Geometry: final body of the model. Coordinates: model frame, mm. A direction names the side the tool comes from. Give positions to 0.01 mm unless a question says otherwise; leave off trailing zeros. Loops run counter-clockwise (first coordinate to the right, second up) from the corner with the lowest first, then second, coordinate; pieces in that order, holes last. Notation, with made-up numbers: (60.25, 78) - (98.25, 78) arc R21 cw to (98.25, 112) - close; hole circle Ø7 at (18.25, -18). An arc over 180 degrees is marked (long way). Answer in a Markdown table with one row per item.
from build123d import *

# Parameters (mm, degrees)
SKETCH1_R           = 5
BOSS_EXTRUDE1_DEPTH = 6.5


with BuildPart() as part:
    # Sketch1 → Boss-Extrude1 (new body)
    with BuildSketch(Plane.XY):
        Polygon((0, -9.814954576), (8.5, -4.907477288), (8.5, 4.907477288), (0, 9.814954576), (-8.5, 4.907477288), (-8.5, -4.907477288), align=None)
        with Locations(Location((0, 0, 0), (0, 0, 180))):
            Circle(SKETCH1_R, mode=Mode.SUBTRACT)
    extrude(amount=BOSS_EXTRUDE1_DEPTH)

    # Sketch3 → Revolve1 (revolve)
    with BuildSketch(Plane(origin=(0, 0, 0), x_dir=(0, 0, -1), z_dir=(0, 1, 0))):
        with BuildLine():
            Line((-6.5, 8.5), (-8.8, 8.5))
            ThreePointArc((-8.8, 8.5), (-9.648528137, 8.148528137), (-10, 7.3))
            Line((-10, 7.3), (-10, 5))
            Line((-10, 5), (-6.5, 5))
            Line((-6.5, 5), (-6.5, 8.5))
        make_face()
    revolve(axis=Axis((0, 0, 0), (0, 0, 1)))

    # Sketch2 → Cut-Revolve1 (revolve, cut)
    with BuildSketch(Plane(origin=(0, 0, 0), x_dir=(0, 0, -1), z_dir=(1, 0, 0)), mode=Mode.PRIVATE) as cut_revolve1_sk:
        Polygon((-6.5, 9.814954576), (-6.5, 8.5), (-5.958333333, 9.814954576), align=None)
        Polygon((-0.541666667, 9.814954576), (0, 9.814954576), (0, 8.5), align=None)
        Polygon((-10, 5), (-9.35, 5), (-10, 5.65), align=None)
        Polygon((0, 5), (-0.65, 5), (0, 5.65), align=None)
    revolve(cut_revolve1_sk.sketch.rotate(Axis((0, 0, 0), (0, 0, 1)), 90), axis=Axis((0, 0, 0), (0, 0, 1)), mode=Mode.SUBTRACT)


solid = part.part
Q1. First-contact query: pin 1 (5 mm diameter, centred on x = -3.5, z = 8, fed in from -Y); pin 2 (1.5 mm diameter, centred on x = 6, y = -6.5, fed in from +Z). Flat tips, straight axial feed; report the tip coordinate or a pass-through.
Check values:
| item | result |
|---|---|
| pin 1 | y = -8.85 |
| pin 2 | z = 9.7 |
Q2. Material intervals for line 1 along X through (y, z) = (2, 4); line 2 along Y through (x, z) = (1.5, 4.5); line 3 along X through (y, z) = (3, 2), sorted ascending.
Check values:
| item | result |
|---|---|
| line 1 | -8.5 to -4.58, 4.58 to 8.5 |
| line 2 | -8.95 to -4.77, 4.77 to 8.95 |
| line 3 | -8.5 to -4, 4 to 8.5 |
Q3. Cut plane A-A (z = 3.5). Output: boundary loops of the cut face in (x, y).
Check values:
| item | result |
|---|---|
| outline | (-8.5, -4.91) - (0, -9.81) - (8.5, -4.91) - (8.5, 4.91) - (0, 9.81) - (-8.5, 4.91) - close; hole circle Ø10 at (0, 0) |
Q4. Reachability of faces 1 (the conical face through (7.627, -4.428, 0.132)), 2 (the cylindrical face through (-4.57, -7.167, 7.666)) from +Z, -Z, +X, -X, +Y, -Y: full face, straight path, thin tool, end or side. Return the list, or none.
Check values:
| item | result |
|---|---|
| face 1 | -Z, +X, -Y |
| face 2 | +Z |
